```python
from build123d import *

# Parameters (mm, degrees)
SKETCH_W     = 66.6
SKETCH_H     = 33.3
SKETCH_R     = 1.5
PAD001_DEPTH = 2
FILLET001_R  = 3
FILLET002_R  = 3


with BuildPart() as part:
    # Sketch → Pad001 (new body)
    with BuildSketch(Plane.XY):
        with BuildLine():
            Line((-58, 21.65), (56, 21.65))
            Line((56, 21.65), (56, -21.65))
            Line((56, -21.65), (-58, -21.65))
            add(Edge.make_bspline(
                [(-58, -21.65), (-93, -21.65), (-93, -5)],
                knots=[0, 0, 0, 1, 1, 1], degree=2))
            Line((-93, -5), (-93, 5))
            add(Edge.make_bspline(
                [(-58, 21.65), (-93, 21.65), (-93, 5)],
                knots=[0, 0, 0, 1, 1, 1], degree=2))
        make_face()
        Rectangle(SKETCH_W, SKETCH_H, mode=Mode.SUBTRACT)
        with Locations((-48, 0)):
            Circle(SKETCH_R, mode=Mode.SUBTRACT)
        with Locations((48, 0)):
            Circle(SKETCH_R, mode=Mode.SUBTRACT)
    extrude(amount=PAD001_DEPTH)

    # Fillet001
    fillet001_edges = [part.edges().sort_by_distance(p)[0] for p in [
        (56, -21.65, 1),
    ]]
    fillet(fillet001_edges, radius=FILLET001_R)

    # Fillet002
    fillet002_edges = [part.edges().sort_by_distance(p)[0] for p in [
        (56, 21.65, 1),
    ]]
    fillet(fillet002_edges, radius=FILLET002_R)


solid = part.part
```
Part model, mm, in its own coordinate system. Coordinates: 2 decimals unless noted, no trailing zeros. Order: outer loops, then holes, each group sorted by start corner. A loop starts at its lowest first (then second) coordinate and runs counter-clockwise, first axis right, second up. Notation, with made-up numbers: (56, 69.5) - (68, 69.5) arc R32 cw to (68, 107.5) - close; hole circle Ø5 at (80.25, 84.5). An arc over 180 degrees is marked (long way). Return JSON: item names as keys, results as strings. Group by question number.
Item 1: Drill centre lines: probe 1 along Y at (x, z) = (-21, 0.9); probe 2 along X at (y, z) = (-3, 0.2); probe 3 along Y at (x, z) = (48, 1.2). Where is each one in solid material? Low to high. Write a range as from..to.
Item 2: Cut at A-A (x = 48). List the corners of the cut face in (y, z).
Item 3: Cut at B-B (y = 0). List the corners of the cut face in (x, z), plus the area to 3 significant figures.
Item 4: Cut at D-D (z = 1.5). State how many separate pieces and enclosed holes the cut face has, plus the area to 3 significant figures.
Item 5: Cut at C-C (x = -6). List the corners of the cut face in (y, z), plus the area to 3 significant figures.
Item 6: Pull direction Y, two halves, no side cores. Call faces 1 (the face through (46.5, 0.07, 0.99)), 2 (the face through (-34, 0, 2)), 3 (the face through (55.14, 20.75, 1.01)): pulls with the +Y half, pulls with the -Y half, needs draft (parallel to the pull), parting line crosses it, or undercut.
Check values:
{
 "1": {"probe 1": "y = -21.65..-16.65, 16.65..21.65", "probe 2": "x = -93..-33.3, 33.3..56", "probe 3": "y = -21.65..-1.5, 1.5..21.65"},
 "2": {"outline": "(-21.65, 0) - (-1.5, 0) - (-1.5, 2) - (-21.65, 2) - close; (1.5, 0) - (21.65, 0) - (21.65, 2) - (1.5, 2) - close"},
 "3": {"outline": "(-93, 0) - (-49.5, 0) - (-49.5, 2) - (-93, 2) - close; (-46.5, 0) - (-33.3, 0) - (-33.3, 2) - (-46.5, 2) - close; (33.3, 0) - (46.5, 0) - (46.5, 2) - (33.3, 2) - close; (49.5, 0) - (56, 0) - (56, 2) - (49.5, 2) - close", "area": "153 mm2"},
 "4": {"separate pieces": "1", "enclosed holes": "3", "area": "4,020 mm2"},
 "5": {"outline": "(-21.65, 0) - (-16.65, 0) - (-16.65, 2) - (-21.65, 2) - close; (16.65, 0) - (21.65, 0) - (21.65, 2) - (16.65, 2) - close", "area": "20.0 mm2"},
 "6": {"face 1": "undercut", "face 2": "needs draft", "face 3": "pulls with the +Y half"}
}
